Job drawing, mm, ordinate dimensions from the low corner. One solid piece. A direction names the side the tool comes from. Coordinates: 2 decimals unless noted, no trailing zeros. Write each loop counter-clockwise with the first axis right and the second up, starting at its lowest first coordinate (ties: lowest second). Pieces come first, ordered by that corner, then holes.
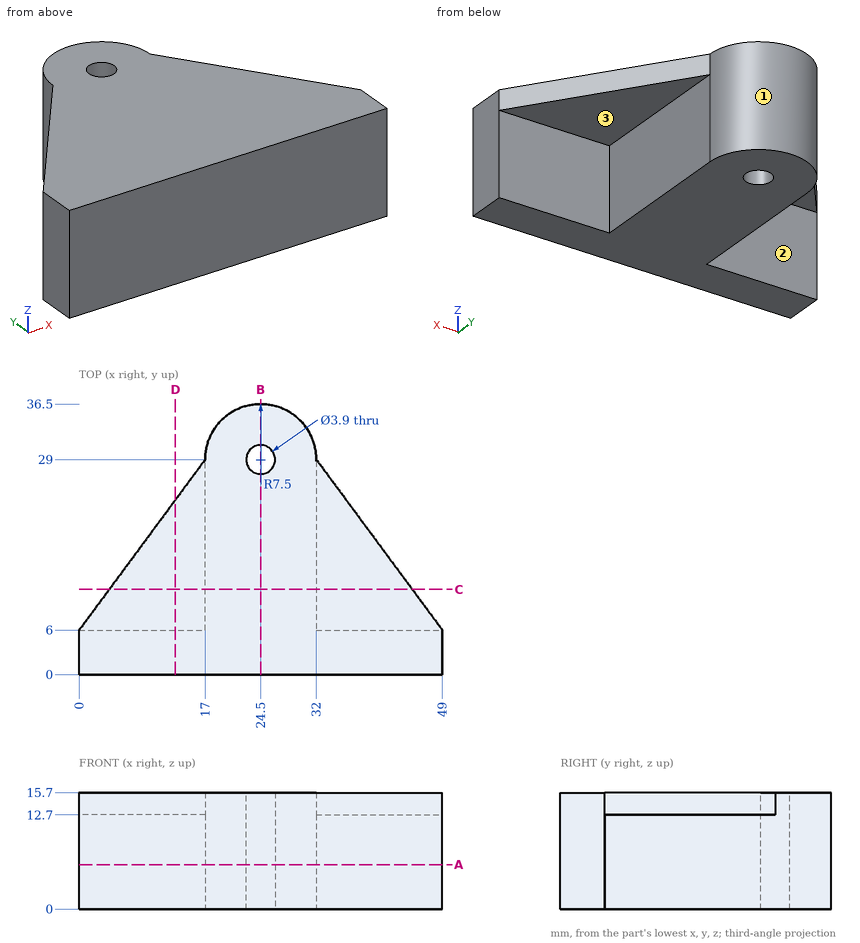
1. Flat gauge pins, fed straight in: pin 1 (5 mm diameter, centred on x = 21.5, z = 2.5, fed in from -Y); pin 2 (6.5 mm diameter, centred on y = 18.5, z = 6, fed in from +X); pin 3 (5 mm diameter, centred on y = 16.5, z = 12.5, fed in from +X); pin 4 (8 mm diameter, centred on y = 14.5, z = 3.5, fed in from -X). Where does each tip first touch, or does it go through?
Computed values:
pin 1: stops at y = 0
pin 2: stops at x = 32
pin 3: stops at x = 43.08
pin 4: stops at x = 17
2. Probe line 1 along Y through (x, z) = (24.5, 7); line 2 along Y through (x, z) = (44.5, 5.5); line 3 along X through (y, z) = (22, 10.5). List the from-to ranges inside material, lowest first.
Computed values:
line 1: y = 0 to 27.05, 30.95 to 36.5
line 2: y = 0 to 6
line 3: x = 17 to 32
3. Saw through at A-A on z = 6. List the corners of the cut face in (x, y).
Computed values:
outline: (0, 0) - (49, 0) - (49, 6) - (32, 6) - (32, 29) arc R7.5 ccw to (17, 29) - (17, 6) - (0, 6) - close; hole circle Ø3.9 at (24.5, 29)
4. Saw through at B-B on x = 24.5. List the corners of the cut face in (y, z), plus the area to 3 significant figures.
Computed values:
outline: (0, 0) - (27.05, 0) - (27.05, 15.7) - (0, 15.7) - close; (30.95, 0) - (36.5, 0) - (36.5, 15.7) - (30.95, 15.7) - close
area: 512 mm2
5. Saw through at D-D on x = 13. List the corners of the cut face in (y, z).
Computed values:
outline: (0, 0) - (6, 0) - (6, 12.7) - (23.59, 12.7) - (23.59, 15.7) - (0, 15.7) - close
6. 3-axis set-ups, long thin cutter, end or side, ignore diameter. For the marked faces 1, 2 and 3: which of +Z, -Z, +X, -X, +Y, -Y reach the whole face in a straight line?
Computed values:
face 1: +Z, -Z, +Y
face 2: -Z, -X, +Y
face 3: -Z, +X, +Y
7. Saw through at C-C on y = 11.5. List the corners of the cut face in (x, z).
Computed values:
outline: (4.07, 12.7) - (17, 12.7) - (17, 0) - (32, 0) - (32, 12.7) - (44.93, 12.7) - (44.93, 15.7) - (4.07, 15.7) - close
